Geometry check sheet. Reference: the model listing, model coordinates, mm. Face numbers are marked on the shaded views. A direction names the side the tool comes from. Round coordinates to 2 decimals unless told otherwise and drop trailing zeros. Order: outer loops, then holes, each group sorted by start corner. A loop starts at its lowest first (then second) coordinate and runs counter-clockwise, first axis right, second up. Notation, with made-up numbers: (-4, -19) - (48, -19) arc R37 ccw to (48, 18) - close; hole circle Ø3 at (21, 22.5). An arc over 180 degrees is marked (long way). One line per question, with ' | ' between items. Start each with the question number.
Q1. Tool access check on the marked faces 1, 2, 3 and 4. Record the directions out of +Z, -Z, +X, -X, +Y, -Y that give a thin tool (end or side, any length) a straight path to the whole face; none if there is none.
Q2. Sectioned sample at A-A, the plane x = 2. Enter the section's corners in (y, z), then the cut area to 3 significant figures.
Q3. Material ranges on line 1 along Z through (x, y) = (12.75, -4.25); line 2 along Z through (x, y) = (17, -4.25); line 3 along X through (y, z) = (3, -1.75), recorded low to high.
Q4. Mould release check, pull along X, two halves, no side actions. Record for the marked faces 5, 6, 7 and 8: +X half, -X half, draft (parallel to the pull), parting line (faces both ways), or undercut.
Q5. Sectioned sample at D-D, the plane z = 8. Enter the section's corners in (x, y), then the cut area to 3 significant figures.
Q6. Gauge pin test, flat ends, axial feed: P1, Ø1.5, axis at x = 11.5, y = 0.5, coming from the +Z side; P2, Ø2.5, axis at y = -1.5, z = 6.5, coming from the +X side; P3, Ø1.5, axis at x = 8, z = -1, coming from the +Y side. Record the tip position at first contact, or that the pin passes through.
Q7. Sectioned sample at B-B, the plane y = 1.25. Enter the section's corners in (x, z).
Q8. Sectioned sample at C-C, the plane z = 6. Enter the section's corners in (x, y), then the cut area to 3 significant figures.
```python
from build123d import *

# Parameters (mm, degrees)
BOSS_EXTRUDE1_DEPTH     = 18
SKETCH2_W               = 9
SKETCH2_H               = 1
CUT_EXTRUDE1_DEPTH      = 18
SKETCH3_R               = 2
CUT_EXTRUDE2_DEPTH      = 3
CUT_EXTRUDE3_DEPTH      = 3
CUT_EXTRUDE3_DEPTH_BACK = 6


with BuildPart() as part:
    # Sketch1 → Boss-Extrude1 (new body)
    with BuildSketch(Plane(origin=(0, 0, 0), x_dir=(0, 0, -1), z_dir=(1, 0, 0))):
        with BuildLine():
            ThreePointArc((-5, 5), (-10, 0), (-5, -5))
            Line((-5, -5), (-5, -2))
            ThreePointArc((-5, -2), (-7, 0), (-5, 2))
            Line((-5, 2), (-5, 5))
        make_face()
        with BuildLine():
            Line((-5, -2), (-5, -5))
            ThreePointArc((-5, -5), (-1.464466094, -3.535533906), (0, 0))
            ThreePointArc((0, 0), (-1.464466094, 3.535533906), (-5, 5))
            Line((-5, 5), (-5, 2))
            ThreePointArc((-5, 2), (-3.585786438, 1.414213562), (-3, 0))
            ThreePointArc((-3, 0), (-3.585786438, -1.414213562), (-5, -2))
        make_face()
        with BuildLine():
            ThreePointArc((-5, 5), (-10, 0), (-5, -5))
            Line((-5, -5), (-5, -2))
            ThreePointArc((-5, -2), (-7, 0), (-5, 2))
            Line((-5, 2), (-5, 5))
        make_face()
        with BuildLine():
            Line((-5, -2), (-5, -5))
            ThreePointArc((-5, -5), (-1.464466094, -3.535533906), (0, 0))
            ThreePointArc((0, 0), (-1.464466094, 3.535533906), (-5, 5))
            Line((-5, 5), (-5, 2))
            ThreePointArc((-5, 2), (-3.585786438, 1.414213562), (-3, 0))
            ThreePointArc((-3, 0), (-3.585786438, -1.414213562), (-5, -2))
        make_face()
        with BuildLine():
            Line((-5, -5), (5, -5))
            Line((5, -5), (5, -3))
            Line((5, -3), (4, -3))
            Line((4, -3), (4, 3))
            Line((4, 3), (5, 3))
            Line((5, 3), (5, 5))
            Line((5, 5), (-5, 5))
            ThreePointArc((-5, 5), (-1.464466094, 3.535533906), (0, 0))
            ThreePointArc((0, 0), (-1.464466094, -3.535533906), (-5, -5))
        make_face()
    extrude(amount=BOSS_EXTRUDE1_DEPTH)

    # Sketch2 → Cut-Extrude1 (cut)
    with BuildSketch(Plane.XZ.offset(5)):
        Polygon((9, 10), (9, 9), (12, 9), (12, 0), (15, -2), (18, -2), (18, 10), align=None)
        with Locations((10.5, -4.5)):
            Rectangle(SKETCH2_W, SKETCH2_H)
    extrude(amount=-CUT_EXTRUDE1_DEPTH, mode=Mode.SUBTRACT)

    # Sketch3 → Cut-Extrude2 (cut)
    with BuildSketch(Plane(origin=(12, 0, 0), x_dir=(0, 0, -1), z_dir=(1, 0, 0))):
        with BuildLine():
            Line((-9, -3), (-5, -3))
            ThreePointArc((-5, -3), (-2, 0), (-5, 3))
            Line((-5, 3), (-9, 3))
            Line((-9, 3), (-9, -3))
        make_face()
        with Locations((-5, 0)):
            Circle(SKETCH3_R, mode=Mode.SUBTRACT)
    extrude(amount=-CUT_EXTRUDE2_DEPTH, mode=Mode.SUBTRACT)

    # Sketch4 → Cut-Extrude3 (cut, two sides)
    with BuildSketch(Plane(origin=(12, 0, 0), x_dir=(0, 0, -1), z_dir=(1, 0, 0))) as cut_extrude3_sk:
        with BuildLine():
            Line((-0.025062814, 0.5), (2, 0.5))
            Line((2, 0.5), (2, 5))
            Line((2, 5), (-5, 5))
            ThreePointArc((-5, 5), (-1.645898034, 3.708099244), (-0.025062814, 0.5))
        make_face()
        with BuildLine():
            Line((-5, -5), (2, -5))
            Line((2, -5), (2, -0.5))
            Line((2, -0.5), (-0.025062814, -0.5))
            ThreePointArc((-0.025062814, -0.5), (-1.645898034, -3.708099244), (-5, -5))
        make_face()
    extrude(amount=CUT_EXTRUDE3_DEPTH, mode=Mode.SUBTRACT)
    extrude(cut_extrude3_sk.sketch, amount=-CUT_EXTRUDE3_DEPTH_BACK, mode=Mode.SUBTRACT)


solid = part.part
```
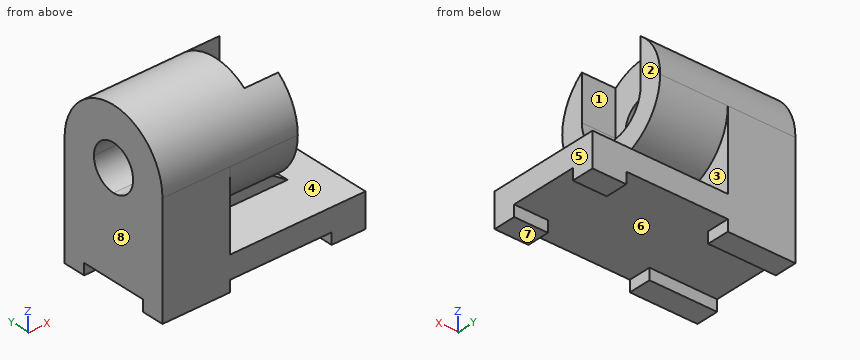
Determined:
1) face 1: +Z, +X | face 2: +Z, +X, +Y, -Y | face 3: +X, +Y | face 4: +X
2) outline: (-5, -5) - (-3, -5) - (-3, -4) - (3, -4) - (3, -5) - (5, -5) - (5, 5) arc R5 ccw to (-5, 5) - close; hole circle Ø4 at (0, 5) | area: 121 mm2
3) line 1: z = -4 to -2 | line 2: z = -5 to -2 | line 3: x = 0 to 6
4) face 5: +X half | face 6: undercut | face 7: draft | face 8: -X half
5) outline: (0, -4) - (12, -4) - (12, -3) - (9, -3) - (9, 3) - (12, 3) - (12, 4) - (0, 4) - close | area: 78.0 mm2
6) P1: stops at z = 2.27 | P2: stops at x = 9 | P3: stops at y = 0.5
7) outline: (0, -4) - (18, -4) - (18, -2) - (6, -2) - (6, 0.16) - (12, 0.16) - (12, 2.27) - (9, 2.27) - (9, 3.44) - (0, 3.44) - close; (0, 6.56) - (9, 6.56) - (9, 9.84) - (0, 9.84) - close
8) outline: (0, -4.9) - (12, -4.9) - (12, -3) - (9, -3) - (9, -1.73) - (0, -1.73) - close; (0, 1.73) - (9, 1.73) - (9, 3) - (12, 3) - (12, 4.9) - (0, 4.9) - close | area: 68.4 mm2
